from build123d import *

# Parameters (mm, degrees)
BOSS_EXTRUDE1_DEPTH = 35
CUT_EXTRUDE1_REACH  = 56.252
SKETCH2_R           = 3
SKETCH2_4_R         = 9
CUT_EXTRUDE2_DEPTH  = 2
CUT_EXTRUDE3_REACH  = 49.804
SKETCH5_R           = 1.7


with BuildPart() as part:
    # Sketch1 → Boss-Extrude1 (new body)
    with BuildSketch(Plane.YZ):
        Polygon((0, -12.79), (35, -12.79), (35, 22.21), (23.81, 22.21), (23.81, 0), (0, 0), align=None)
    extrude(amount=BOSS_EXTRUDE1_DEPTH)

    # Sketch2 → Cut-Extrude1 (cut, up to next)
    with BuildSketch(Plane.XY, mode=Mode.PRIVATE) as cut_extrude1_sk1:
        with Locations((17.5, 11.905)):
            Circle(SKETCH2_R)
    cut_extrude1_tool1 = extrude(cut_extrude1_sk1.sketch, amount=-CUT_EXTRUDE1_REACH, mode=Mode.PRIVATE) & part.part
    add(cut_extrude1_tool1.solids().sort_by_distance((17.5, 11.905, 0))[0], mode=Mode.SUBTRACT)

    # Sketch2_4 → Cut-Extrude2 (cut)
    with BuildSketch(Plane.XY):
        with Locations((17.5, 11.905)):
            Circle(SKETCH2_4_R)
    extrude(amount=-CUT_EXTRUDE2_DEPTH, mode=Mode.SUBTRACT)

    # Sketch5 → Cut-Extrude3 (cut, up to next)
    with BuildSketch(Plane.XZ.offset(-23.81), mode=Mode.PRIVATE) as cut_extrude3_sk1:
        with Locations(Location((5, 17.21, 0), (0, 0, 270))):
            Circle(SKETCH5_R)
    cut_extrude3_tool1 = extrude(cut_extrude3_sk1.sketch, amount=-CUT_EXTRUDE3_REACH, mode=Mode.PRIVATE) & part.part
    # Sketch5 → Cut-Extrude3 (cut, up to next)
    with BuildSketch(Plane.XZ.offset(-23.81), mode=Mode.PRIVATE) as cut_extrude3_sk2:
        with Locations(Location((30, 17.21, 0), (0, 0, 270))):
            Circle(SKETCH5_R)
    cut_extrude3_tool2 = extrude(cut_extrude3_sk2.sketch, amount=-CUT_EXTRUDE3_REACH, mode=Mode.PRIVATE) & part.part
    # Sketch5 → Cut-Extrude3 (cut, up to next)
    with BuildSketch(Plane.XZ.offset(-23.81), mode=Mode.PRIVATE) as cut_extrude3_sk3:
        with Locations(Location((30, 5, 0), (0, 0, 270))):
            Circle(SKETCH5_R)
    cut_extrude3_tool3 = extrude(cut_extrude3_sk3.sketch, amount=-CUT_EXTRUDE3_REACH, mode=Mode.PRIVATE) & part.part
    # Sketch5 → Cut-Extrude3 (cut, up to next)
    with BuildSketch(Plane.XZ.offset(-23.81), mode=Mode.PRIVATE) as cut_extrude3_sk4:
        with Locations(Location((5, 5, 0), (0, 0, 270))):
            Circle(SKETCH5_R)
    cut_extrude3_tool4 = extrude(cut_extrude3_sk4.sketch, amount=-CUT_EXTRUDE3_REACH, mode=Mode.PRIVATE) & part.part
    add(cut_extrude3_tool1.solids().sort_by_distance((5, 23.81, 17.21))[0], mode=Mode.SUBTRACT)
    add(cut_extrude3_tool2.solids().sort_by_distance((30, 23.81, 17.21))[0], mode=Mode.SUBTRACT)
    add(cut_extrude3_tool3.solids().sort_by_distance((30, 23.81, 5))[0], mode=Mode.SUBTRACT)
    add(cut_extrude3_tool4.solids().sort_by_distance((5, 23.81, 5))[0], mode=Mode.SUBTRACT)


solid = part.part
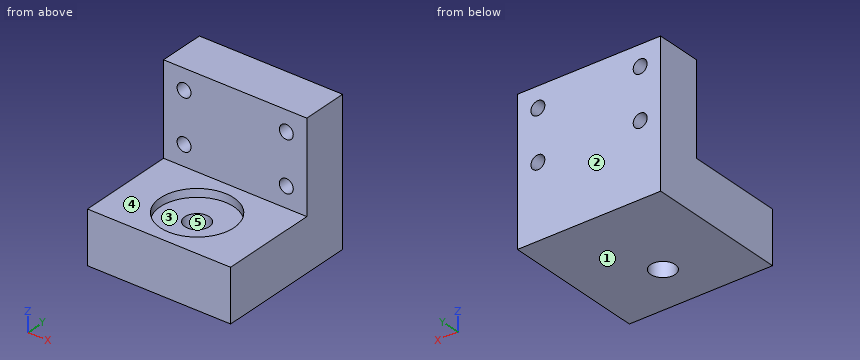
Source: CAD feature listing. Evaluate the final solid. Frame: model axes, mm. Face numbers are marked on the shaded views. A direction names the side the tool comes from. Give positions to 0.01 mm unless a question says otherwise; leave off trailing zeros. Write each loop counter-clockwise with the first axis right and the second up, starting at its lowest first coordinate (ties: lowest second). Pieces come first, ordered by that corner, then holes. Notation, with made-up numbers: M 70.5,-23.5 L 103.5,-23.5 A22 ccw 103.5,-14.5 Z; hole C 7,69 d7. An arc over 180 degrees is marked long. Return JSON: item names as keys, results as strings. Group by question number.
1) Material intervals for line 1 along X through (y, z) = (27.75, 5); line 2 along Y through (x, z) = (17.5, -7) (3 decimals); line 3 along X through (y, z) = (33, 4.5), sorted ascending. Write a range as [from, to].
2) Cut plane B-B, the plane z = 17.21. Output: boundary loops of the cut face in (x, y), plus the area to 3 significant figures.
3) Cut plane C-C, the plane y = 13. Output: boundary loops of the cut face in (x, z).
4) Set-up query: the marked faces 4 and 5. Return all of +Z, -Z, +X, -X, +Y, -Y with unobstructed straight access to the full face (end or side cutting, diameter ignored); none if empty.
5) Pin query (flat end, axial travel): P1, Ø7, axis at x = 20, y = 7.5, coming from the +Z side; P2, Ø5.5, axis at x = 5, z = 5, coming from the -Y side; P3, Ø8, axis at x = 14, y = 18.5, coming from the +Z side; P4, Ø5, axis at y = 19.5, z = 6, coming from the -X side. Return the tip coordinate at first contact, or that it passes through.
6) Cut plane A-A, the plane x = 17.5. Output: boundary loops of the cut face in (y, z) (3 decimals), plus the area to 3 significant figures.
7) Pull-direction query (Y, two-part tool) for the marked faces 1, 2 and 3; classes: pulls with the +Y half, pulls with the -Y half, needs draft (parallel to the pull), parting line crosses it, or undercut.
8) Cut plane D-D, the plane x = 5. Output: boundary loops of the cut face in (y, z), plus the area to 3 significant figures.
Recorded:
{
 "1": {"line 1": "x = [0, 3.3], [6.7, 28.3], [31.7, 35]", "line 2": "y = [0, 8.905], [14.905, 35]", "line 3": "x = [0, 3.38], [6.62, 28.38], [31.62, 35]"},
 "2": {"outline": "M 0,23.81 L 3.3,23.81 L 3.3,35 L 0,35 Z; M 6.7,23.81 L 28.3,23.81 L 28.3,35 L 6.7,35 Z; M 31.7,23.81 L 35,23.81 L 35,35 L 31.7,35 Z", "area": "316 mm²"},
 "3": {"outline": "M 0,-12.79 L 14.71,-12.79 L 14.71,-2 L 8.57,-2 L 8.57,0 L 0,0 Z; M 20.29,-12.79 L 35,-12.79 L 35,0 L 26.43,0 L 26.43,-2 L 20.29,-2 Z"},
 "4": {"face 4": "+Z, +X, -X, -Y", "face 5": "+Z, -Z"},
 "5": {"P1": "stops at z = -2", "P2": "stops at y = 23.81", "P3": "stops at z = 0", "P4": "passes through"},
 "6": {"outline": "M 0,-12.79 L 8.905,-12.79 L 8.905,-2 L 2.905,-2 L 2.905,0 L 0,0 Z; M 14.905,-12.79 L 35,-12.79 L 35,22.21 L 23.81,22.21 L 23.81,0 L 20.905,0 L 20.905,-2 L 14.905,-2 Z", "area": "595 mm²"},
 "7": {"face 1": "needs draft", "face 2": "pulls with the +Y half", "face 3": "undercut"},
 "8": {"outline": "M 0,-12.79 L 35,-12.79 L 35,3.3 L 23.81,3.3 L 23.81,0 L 0,0 Z; M 23.81,6.7 L 35,6.7 L 35,15.51 L 23.81,15.51 Z; M 23.81,18.91 L 35,18.91 L 35,22.21 L 23.81,22.21 Z", "area": "620 mm²"}
}
